Check sheet for the modelled part. Datum: model origin and axes. Units: mm. A direction names the side the tool comes from. Round coordinates to 2 decimals unless told otherwise and drop trailing zeros. Loops run counter-clockwise (first coordinate to the right, second up) from the corner with the lowest first, then second, coordinate; pieces in that order, holes last. Notation, with made-up numbers: (-1.5, -20.5) -> (33.5, -20.5) arc R25 ccw to (33.5, 12.5) -> close; hole circle Ø8 at (-18, -2). An arc over 180 degrees is marked (long way). One line per question, with ' | ' between items.
```python
from build123d import *

# Parameters (mm, degrees)
SKETCH1_R               = 8
SKETCH1_R_2             = 4
BOSS_EXTRUDE1_DEPTH     = 13
CUT_EXTRUDE1_REACH      = 19.234
CUT_EXTRUDE1_END_RADIUS = 8
SKETCH2_R               = 2
CUT_EXTRUDE2_REACH      = 19.234
CUT_EXTRUDE2_END_RADIUS = 8
SKETCH3_R               = 2
SKETCH4_R               = 16
SKETCH4_R_2             = 4
BOSS_EXTRUDE2_DEPTH     = 3
CUT_EXTRUDE3_REACH      = 26.739
SKETCH5_R               = 2
FILLET1_R               = 0.5


with BuildPart() as part:
    # Sketch1 → Boss-Extrude1 (new body)
    with BuildSketch(Plane(origin=(0, 0, 0), x_dir=(1, 0, 0), z_dir=(0, 1, 0))):
        with Locations(Location((0, 0, 0), (0, 0, 90))):
            Circle(SKETCH1_R)
        with Locations(Location((0, 0, 0), (0, 0, 90))):
            Circle(SKETCH1_R_2, mode=Mode.SUBTRACT)
    extrude(amount=BOSS_EXTRUDE1_DEPTH)

    # Cut-Extrude1: up to this cylinder (the profile starts inside it)
    cut_extrude1_end = Plane(origin=(0, 8.5, 0), z_dir=(0, -1, 0)) * Cylinder(CUT_EXTRUDE1_END_RADIUS, 55.468, mode=Mode.PRIVATE)
    # Sketch2 → Cut-Extrude1 (cut, up to the surface)
    with BuildSketch(Plane.XY, mode=Mode.PRIVATE) as cut_extrude1_sk1:
        with Locations((0, 8.5)):
            Circle(SKETCH2_R)
    cut_extrude1_tool1 = extrude(cut_extrude1_sk1.sketch, amount=-CUT_EXTRUDE1_REACH, mode=Mode.PRIVATE) & cut_extrude1_end
    add(cut_extrude1_tool1.solids().sort_by_distance((0, 8.5, 0))[0], mode=Mode.SUBTRACT)

    # Cut-Extrude2: up to this cylinder (the profile starts inside it)
    cut_extrude2_end = Plane(origin=(0, 8.5, 0), z_dir=(0, -1, 0)) * Cylinder(CUT_EXTRUDE2_END_RADIUS, 55.468, mode=Mode.PRIVATE)
    # Sketch3 → Cut-Extrude2 (cut, up to the surface)
    with BuildSketch(Plane(origin=(0, 0, 0), x_dir=(0, 0, -1), z_dir=(1, 0, 0)), mode=Mode.PRIVATE) as cut_extrude2_sk1:
        with Locations((0, 8.5)):
            Circle(SKETCH3_R)
    cut_extrude2_tool1 = extrude(cut_extrude2_sk1.sketch, amount=-CUT_EXTRUDE2_REACH, mode=Mode.PRIVATE) & cut_extrude2_end
    add(cut_extrude2_tool1.solids().sort_by_distance((0, 8.5, 0))[0], mode=Mode.SUBTRACT)

    # Sketch4 → Boss-Extrude2 (add)
    with BuildSketch(Plane.XZ):
        with Locations(Location((0, 0, 0), (0, 0, 270))):
            Circle(SKETCH4_R)
        with Locations(Location((0, 0, 0), (0, 0, 90))):
            Circle(SKETCH4_R_2, mode=Mode.SUBTRACT)
    extrude(amount=-BOSS_EXTRUDE2_DEPTH)

    # Sketch5 → Cut-Extrude3 (cut, up to next)
    with BuildSketch(Plane(origin=(0, 3, 0), x_dir=(1, 0, 0), z_dir=(0, 1, 0)), mode=Mode.PRIVATE) as cut_extrude3_sk1:
        with Locations(Location((-12, 0, 0), (0, 0, 270))):
            Circle(SKETCH5_R)
    cut_extrude3_tool1 = extrude(cut_extrude3_sk1.sketch, amount=-CUT_EXTRUDE3_REACH, mode=Mode.PRIVATE) & part.part
    # Sketch5 → Cut-Extrude3 (cut, up to next)
    with BuildSketch(Plane(origin=(0, 3, 0), x_dir=(1, 0, 0), z_dir=(0, 1, 0)), mode=Mode.PRIVATE) as cut_extrude3_sk2:
        with Locations(Location((0, 12, 0), (0, 0, 270))):
            Circle(SKETCH5_R)
    cut_extrude3_tool2 = extrude(cut_extrude3_sk2.sketch, amount=-CUT_EXTRUDE3_REACH, mode=Mode.PRIVATE) & part.part
    # Sketch5 → Cut-Extrude3 (cut, up to next)
    with BuildSketch(Plane(origin=(0, 3, 0), x_dir=(1, 0, 0), z_dir=(0, 1, 0)), mode=Mode.PRIVATE) as cut_extrude3_sk3:
        with Locations(Location((12, 0, 0), (0, 0, 270))):
            Circle(SKETCH5_R)
    cut_extrude3_tool3 = extrude(cut_extrude3_sk3.sketch, amount=-CUT_EXTRUDE3_REACH, mode=Mode.PRIVATE) & part.part
    # Sketch5 → Cut-Extrude3 (cut, up to next)
    with BuildSketch(Plane(origin=(0, 3, 0), x_dir=(1, 0, 0), z_dir=(0, 1, 0)), mode=Mode.PRIVATE) as cut_extrude3_sk4:
        with Locations(Location((0, -12, 0), (0, 0, 270))):
            Circle(SKETCH5_R)
    cut_extrude3_tool4 = extrude(cut_extrude3_sk4.sketch, amount=-CUT_EXTRUDE3_REACH, mode=Mode.PRIVATE) & part.part
    add(cut_extrude3_tool1.solids().sort_by_distance((-12, 3, 0))[0], mode=Mode.SUBTRACT)
    add(cut_extrude3_tool2.solids().sort_by_distance((0, 3, -12))[0], mode=Mode.SUBTRACT)
    add(cut_extrude3_tool3.solids().sort_by_distance((12, 3, 0))[0], mode=Mode.SUBTRACT)
    add(cut_extrude3_tool4.solids().sort_by_distance((0, 3, 12))[0], mode=Mode.SUBTRACT)

    # Fillet1
    fillet1_edges = [part.edges().sort_by_distance(p)[0] for p in [
        (0, 3, 16),
        (0, 13, 8),
    ]]
    fillet(fillet1_edges, radius=FILLET1_R)


solid = part.part
```
(1) Set-up check for faces 1 (the face through (-1.2, 1.5, -13.6)), 2 (the face through (-7, 3, -7)): record each of +Z, -Z, +X, -X, +Y, -Y from which the full face is reachable in a straight line by a thin tool's end or side.
Answer:
face 1: +Y, -Y | face 2: +Y
(2) Sectioned sample at D-D, the plane y = 11.75. Record the cut outline in (x, z).
Answer:
outline: circle Ø16 at (0, 0); hole circle Ø8 at (0, 0)
(3) Sectioned sample at B-B, the plane y = 1.25. Record the cut outline in (x, z), and give its area (3 significant figures).
Answer:
outline: circle Ø32 at (0, 0); hole circle Ø4 at (-12, 0); hole circle Ø8 at (0, 0); hole circle Ø4 at (0, -12); hole circle Ø4 at (0, 12); hole circle Ø4 at (12, 0) | area: 704 mm2
(4) Scan lines: probe 1 along X at (y, z) = (2.45, 0); probe 2 along X at (y, z) = (2.25, -0.5); probe 3 along Z at (x, y) = (0, 9). Record each from-to range of solid material in increasing order.
Answer:
probe 1: x = -16 to -14, -10 to -4, 4 to 10, 14 to 16 | probe 2: x = -15.99 to -13.94, -10.06 to -3.97, 3.97 to 10.06, 13.94 to 15.99 | probe 3: z = 4 to 8
(5) Sectioned sample at A-A, the plane x = 0. Record the cut outline in (y, z), and give its area (3 significant figures).
Answer:
outline: (0, -16) -> (2.5, -16) arc R0.5 ccw to (3, -15.5) -> (3, -14) -> (0, -14) -> close; (0, -10) -> (3, -10) -> (3, -8) -> (6.5, -8) -> (6.5, -4) -> (0, -4) -> close; (0, 4) -> (13, 4) -> (13, 7.5) arc R0.5 ccw to (12.5, 8) -> (3, 8) -> (3, 10) -> (0, 10) -> close; (0, 14) -> (3, 14) -> (3, 15.5) arc R0.5 ccw to (2.5, 16) -> (0, 16) -> close; (10.5, -8) -> (12.5, -8) arc R0.5 ccw to (13, -7.5) -> (13, -4) -> (10.5, -4) -> close | area: 112 mm2
(6) Mould release check, pull along Z, two halves, no side actions. Record for faces 3 (the face through (-5.704, 6.726, -0.923)), 4 (the face through (0.923, 6.726, -5.7)), 5 (the face through (7.81, 7.68, 1.73)): +Z half, -Z half, draft (parallel to the pull), parting line (faces both ways), or undercut.
Answer:
face 3: undercut | face 4: draft | face 5: parting line
(7) Sectioned sample at C-C, the plane y = 10. Record the cut outline in (x, z), and give its area (3 significant figures).
Answer:
outline: (-7.89, -1.32) arc R8 ccw to (-1.32, -7.89) -> (-1.32, -3.77) arc R4 cw to (-3.77, -1.32) -> close; (-7.89, 1.32) -> (-3.77, 1.32) arc R4 cw (long way) to (1.32, -3.77) -> (1.32, -7.89) arc R8 ccw (long way) to start | area: 129 mm2
(8) Go/stop test with flat-tipped pins: pin 1 (4.5 mm diameter, centred on x = -12, z = 0, fed in from +Y); pin 2 (2.5 mm diameter, centred on y = 8.5, z = 0, fed in from +X); pin 3 (2.5 mm diameter, centred on x = 0, y = 8.5, fed in from +Z); pin 4 (5 mm diameter, centred on x = 12, z = 0, fed in from -Y). Record where each tip stops, or that it passes through.
Answer:
pin 1: stops at y = 3 | pin 2: stops at x = 8 | pin 3: stops at z = 8 | pin 4: stops at y = 0
